CAD build for the part. Positions are in the model's coordinates, mm. Face numbers are marked on the shaded views. A direction names the side the tool comes from. Round coordinates to 2 decimals unless told otherwise and drop trailing zeros. Write each loop counter-clockwise with the first axis right and the second up, starting at its lowest first coordinate (ties: lowest second). Pieces come first, ordered by that corner, then holes. Notation, with made-up numbers: (44.5, -11) -> (99.5, -11) arc R16 ccw to (99.5, 7) -> close; hole circle Ø5 at (-36, 27). An arc over 180 degrees is marked (long way). Put each result on its own line as item: value. Start each with the question number.
1. Saw through at A-A on z = 0. List the corners of the cut face in (x, y).
2. 3-axis set-ups, long thin cutter, end or side, ignore diameter. For the marked faces 5, 6, 7, 8 and 9: which of +Z, -Z, +X, -X, +Y, -Y reach the whole face in a straight line?
3. Drill centre lines: line 1 (Y direction, x = 2.5, z = 0); line 2 (Y direction, x = 15, z = 9); line 3 (Z direction, x = 19, y = 67). Where is each one in solid material? Low to high. Write a range as from..to.
4. Saw through at D-D on z = -13. List the corners of the cut face in (x, y).
5. Saw through at C-C on y = 61. List the corners of the cut face in (x, z).
6. Pull direction X, two halves, no side cores. Call the marked faces 1, 2, 3 and 4: pulls with the +X half, pulls with the -X half, needs draft (parallel to the pull), parting line crosses it, or undercut.
7. Saw through at B-B on x = 15. List the corners of the cut face in (y, z), and give its area (3 significant figures).
8. Flat gauge pins, fed straight in: P1, Ø7, axis at y = 55.5, z = 12, coming from the +X side; P2, Ø1, axis at x = 8.5, z = -4.5, coming from the +Y side; P3, Ø4, axis at y = 13.5, z = -6, coming from the +X side. Where does each tip first touch, or does it go through?
from build123d import *

# Parameters (mm, degrees)
BOSS_EXTRUDE1_DEPTH              = 15
BOSS_EXTRUDE2_START              = 6
SKETCH1_5_R                      = 6
BOSS_EXTRUDE2_DEPTH              = 9
BOSS_EXTRUDE5_START              = -15
SKETCH1_8_R                      = 6
BOSS_EXTRUDE5_DEPTH              = 9
FILLET1_RADIUS                   = 15
FILLET1_LENGTH                   = 9
FILLET2_RADIUS                   = 15
FILLET2_LENGTH                   = 9
F_12_0MM_DOWEL_HOLE1_D           = 12
F_12_0MM_DOWEL_HOLE1_ON_FACE_2_D = 12
FILLET3_R                        = 1.5


with BuildPart() as part:
    # Sketch1 → Boss-Extrude1 (new, symmetric)
    with BuildSketch(Plane.XY):
        Polygon((30, 45), (0, 45), (0, 0), (9, 0), (9, 36), (60, 36), (60, 45), align=None)
    extrude(amount=BOSS_EXTRUDE1_DEPTH, both=True)

    # Sketch1<5> → Boss-Extrude2 (add)
    with BuildSketch(Plane.XY.offset(BOSS_EXTRUDE2_START)):
        with BuildLine():
            ThreePointArc((30, 60), (15, 75), (0, 60))
            Line((0, 60), (0, 45))
            Line((0, 45), (30, 45))
            Line((30, 45), (30, 60))
        make_face()
        with Locations((15, 60)):
            Circle(SKETCH1_5_R, mode=Mode.SUBTRACT)
    extrude(amount=BOSS_EXTRUDE2_DEPTH)

    # Sketch1<8> → Boss-Extrude5 (add)
    with BuildSketch(Plane.XY.offset(BOSS_EXTRUDE5_START)):
        with BuildLine():
            ThreePointArc((30, 60), (15, 75), (0, 60))
            Line((0, 60), (0, 45))
            Line((0, 45), (30, 45))
            Line((30, 45), (30, 60))
        make_face()
        with Locations((15, 60)):
            Circle(SKETCH1_8_R, mode=Mode.SUBTRACT)
    extrude(amount=BOSS_EXTRUDE5_DEPTH)

    # Fillet1: full round fillet: the end face becomes a half cylinder, R = half its width
    fillet1_face = Plane((60, 40.5, 0), x_dir=(0, -1, 0), z_dir=(1, 0, 0))  # on the end face: x along it, z out of the body
    fillet1_slab = fillet1_face.offset(-FILLET1_RADIUS / 2) * Box(FILLET1_LENGTH, 2 * FILLET1_RADIUS, FILLET1_RADIUS, mode=Mode.PRIVATE)  # the body's end, R deep
    fillet1_round = Plane((45, 40.5, 0), x_dir=(1, 0, 0), z_dir=(0, -1, 0)) * Cylinder(FILLET1_RADIUS, FILLET1_LENGTH, mode=Mode.PRIVATE)  # its axis R under the face
    add(fillet1_slab - fillet1_round, mode=Mode.SUBTRACT)

    # Fillet2: full round fillet: the end face becomes a half cylinder, R = half its width
    fillet2_face = Plane((4.5, 0, 0), x_dir=(-1, 0, 0), z_dir=(0, -1, 0))  # on the end face: x along it, z out of the body
    fillet2_slab = fillet2_face.offset(-FILLET2_RADIUS / 2) * Box(FILLET2_LENGTH, 2 * FILLET2_RADIUS, FILLET2_RADIUS, mode=Mode.PRIVATE)  # the body's end, R deep
    fillet2_round = Plane((4.5, 15, 0), x_dir=(0, -1, 0), z_dir=(-1, 0, 0)) * Cylinder(FILLET2_RADIUS, FILLET2_LENGTH, mode=Mode.PRIVATE)  # its axis R under the face
    add(fillet2_slab - fillet2_round, mode=Mode.SUBTRACT)

    # Ø12.0mm Dowel Hole1 (through all)
    with Locations(Plane(origin=(45, 45, 0), x_dir=(1, 0, 0), z_dir=(0, 1, 0))):
        with Locations((0, 0)):
            Hole(F_12_0MM_DOWEL_HOLE1_D / 2)

    # Ø12.0mm Dowel Hole1 on face 2 (through all)
    with Locations(Plane(origin=(9, 15, 0), x_dir=(0, 0, 1), z_dir=(1, 0, 0))):
        with Locations((0, 0)):
            Hole(F_12_0MM_DOWEL_HOLE1_ON_FACE_2_D / 2)

    # Fillet3
    fillet3_edges = [part.edges().sort_by_distance(p)[0] for p in [
        (9, 36, 0),
        (30, 45, 10.5),
        (30, 45, -10.5),
    ]]
    fillet(fillet3_edges, radius=FILLET3_R)


solid = part.part
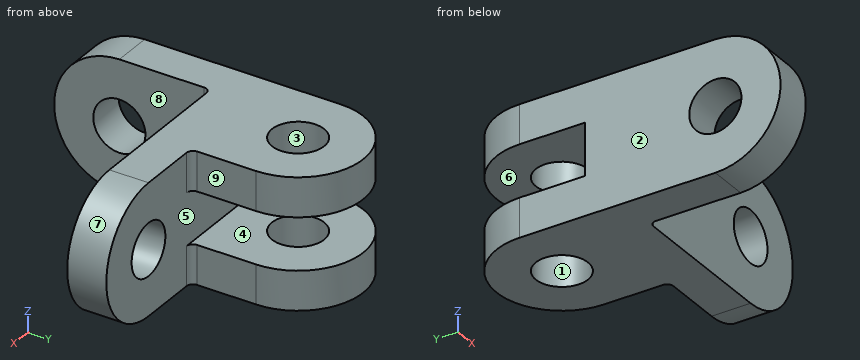
Return value:
1. outline: (0, 0) -> (9, 0) -> (9, 9) -> (0, 9) -> close; (0, 21) -> (9, 21) -> (9, 34.5) arc R1.5 cw to (10.5, 36) -> (39, 36) -> (39, 45) -> (0, 45) -> close; (51, 36) -> (60, 36) -> (60, 45) -> (51, 45) -> close
2. face 5: +X, +Y
2. face 6: +X, -X, +Y
2. face 7: +X, +Y, -Y
2. face 8: +Z, -Z, +X, -Y
2. face 9: +Z, -Z, +X, +Y
3. line 1: y = 0..9, 21..45
3. line 2: y = 36..54, 66..75
3. line 3: z = -15..-6, 6..15
4. outline: (0, 7.52) -> (9, 7.52) -> (9, 34.5) arc R1.5 cw to (10.5, 36) -> (52.48, 36) -> (52.48, 45) -> (31.5, 45) arc R1.5 cw to (30, 46.5) -> (30, 60) arc R15 ccw to (0, 60) -> close; hole circle Ø12 at (15, 60)
5. outline: (0.03, -15) -> (9.08, -15) -> (9.08, -6) -> (0.03, -6) -> close; (0.03, 6) -> (9.08, 6) -> (9.08, 15) -> (0.03, 15) -> close; (20.92, -15) -> (29.97, -15) -> (29.97, -6) -> (20.92, -6) -> close; (20.92, 6) -> (29.97, 6) -> (29.97, 15) -> (20.92, 15) -> close
6. face 1: undercut
6. face 2: pulls with the -X half
6. face 3: undercut
6. face 4: needs draft
7. outline: (36, -15) -> (54, -15) -> (54, -6) -> (45, -6) -> (45, 6) -> (54, 6) -> (54, 15) -> (36, 15) -> close; (66, -15) -> (75, -15) -> (75, -6) -> (66, -6) -> close; (66, 6) -> (75, 6) -> (75, 15) -> (66, 15) -> close
7. area: 594 mm^2
8. P1: stops at x = 30
8. P2: stops at y = 45
8. P3: stops at x = 9
